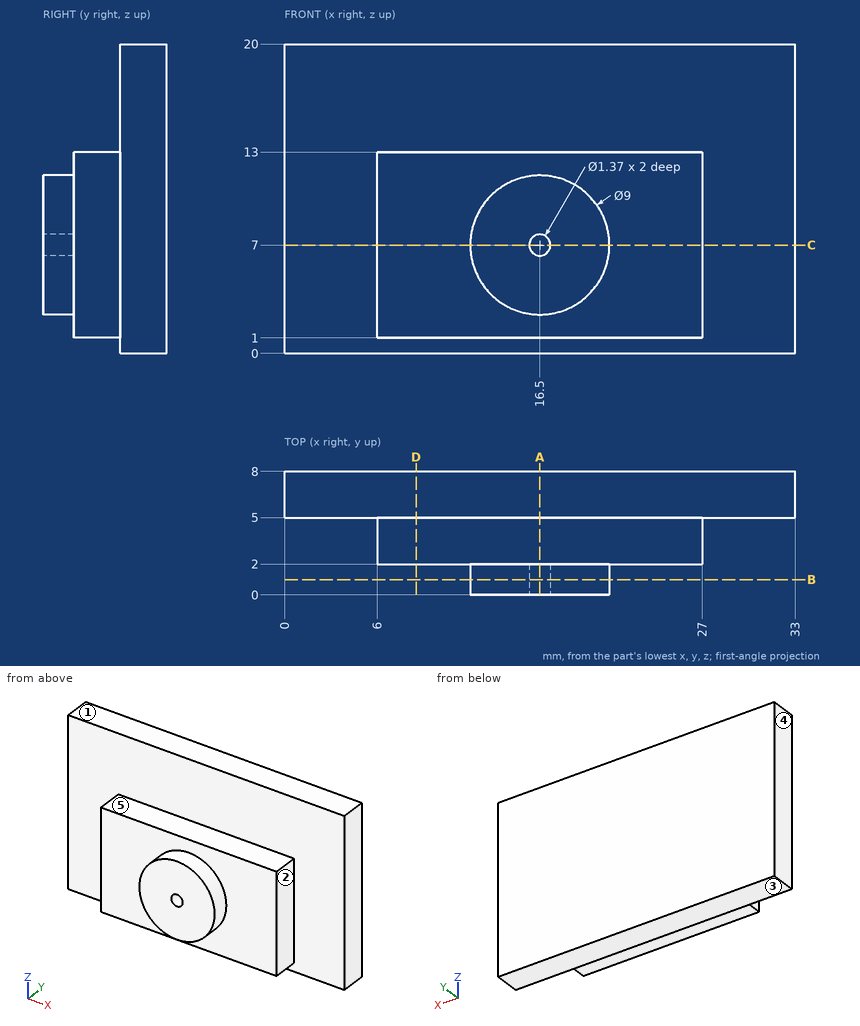
Geometry: see drawing. Coordinates: mm, zero at the bounding-box minimum. A direction names the side the tool comes from. Give positions to 0.01 mm unless a question says otherwise; leave off trailing zeros. Loops run counter-clockwise (first coordinate to the right, second up) from the corner with the lowest first, then second, coordinate; pieces in that order, holes last. Notation, with made-up numbers: (-11.5, 26) - (17.5, 26) arc R18 ccw to (17.5, 38) - close; hole circle Ø10 at (21.5, 72). An arc over 180 degrees is marked (long way). One line per question, with ' | ' between items. Start each with the question number.
(1) Pull-direction query (Z, two-part tool) for the marked faces 1, 2 and 3; classes: released by +Z, released by -Z, zero draft, split by the parting line, or undercut.
(2) Section query B-B on y = 1. Return loops of the section in (x, z) (3 decimals), then the cut area to 3 significant figures.
(3) Section query D-D on x = 8.5. Return loops of the section in (y, z).
(4) Contact query for flat-ended pins moving along their axis: pin 1 (1.5 mm diameter, centred on x = 16, y = 3.5, fed in from -Z); pin 2 (0.9 mm diameter, centred on y = 3, z = 10, fed in from +X); pin 3 (1.5 mm diameter, centred on y = 3.5, z = 7.5, fed in from -X). Output: stop coordinate, or through.
(5) Section query C-C on z = 7. Return loops of the section in (x, y) (3 decimals), then the cut area to 3 significant figures.
(6) Reachability of the marked faces 4 and 5 from +Z, -Z, +X, -X, +Y, -Y: full face, straight path, thin tool, end or side. Return the list, or none.
(7) Ray query, line 1 (Z direction, x = 16.5, y = 0.4) (3 decimals); line 2 (X direction, y = 2.5, z = 12.75); line 3 (Z direction, x = 18.5, y = 2.75). Return the intervals inside material, ascending. Write a range as from..to.
(8) Section query A-A on x = 16.5. Return loops of the section in (y, z) (3 decimals).
The answers:
1) face 1: released by +Z | face 2: zero draft | face 3: released by -Z
2) outline: circle Ø9 at (16.5, 7); hole circle Ø1.37 at (16.5, 7) | area: 62.1 mm2
3) outline: (2, 1) - (5, 1) - (5, 0) - (8, 0) - (8, 20) - (5, 20) - (5, 13) - (2, 13) - close
4) pin 1: z = 1 | pin 2: x = 27 | pin 3: x = 6
5) outline: (0, 5) - (6, 5) - (6, 2) - (12, 2) - (12, 0) - (15.815, 0) - (15.815, 2) - (17.185, 2) - (17.185, 0) - (21, 0) - (21, 2) - (27, 2) - (27, 5) - (33, 5) - (33, 8) - (0, 8) - close | area: 177 mm2
6) face 4: +Z, -Z, -X, +Y, -Y | face 5: +Z, +X, -X, -Y
7) line 1: 2.5..6.315, 7.685..11.5 | line 2: 6..27 | line 3: 1..13
8) outline: (0, 2.5) - (2, 2.5) - (2, 1) - (5, 1) - (5, 0) - (8, 0) - (8, 20) - (5, 20) - (5, 13) - (2, 13) - (2, 11.5) - (0, 11.5) - (0, 7.685) - (2, 7.685) - (2, 6.315) - (0, 6.315) - close
